from build123d import *

# Parameters (mm, degrees)
F0_W     = 609.6
F0_H     = 838.2
F1_DEPTH = 584.2
F2_DEPTH = 2.032
F3_W     = 609.6
F3_H     = 406.4
F4_DEPTH = 44.45
F5_W     = 609.6
F5_H     = 76.2
F6_DEPTH = 12.7


with BuildPart() as f1:
    # F0 (on Front) → F1 (new body)
    with BuildSketch(Plane.XZ):
        with Locations((-304.8, 419.1)):
            Rectangle(F0_W, F0_H)
    extrude(amount=-F1_DEPTH)

    # F0 (on Front) → F2 (join)
    with BuildSketch(Plane.XZ):
        Polygon((0, 838.2), (0, 0), (19.05, 0), (19.05, 857.25), (-628.65, 857.25), (-628.65, 0), (-609.6, 0), (-609.6, 838.2), align=None)
    extrude(amount=-F2_DEPTH)

    # F3 (on face) → F4 (join)
    with BuildSketch(Plane.XZ):
        with Locations((-304.8, 635)):
            Rectangle(F3_W, F3_H)
        with Locations((-304.8, 203.2)):
            Rectangle(F3_W, F3_H)
    extrude(amount=F4_DEPTH)

    # F5 (on face) → F6 (join)
    with BuildSketch(Plane(origin=(0, 0, 0), x_dir=(1, 0, 0), z_dir=(0, 0, -1))):
        with Locations((-304.8, -114.060853)):
            Rectangle(F5_W, F5_H)
        with Locations((-304.8, -331.216)):
            Rectangle(F5_W, F5_H)
    extrude(amount=F6_DEPTH)


solid = f1.part
Check sheet for the modelled part. Datum: model origin and axes. Units: mm. A direction names the side the tool comes from. Give positions to 0.01 mm unless a question says otherwise; leave off trailing zeros. Loops run counter-clockwise (first coordinate to the right, second up) from the corner with the lowest first, then second, coordinate; pieces in that order, holes last. Notation, with made-up numbers: M -13.75,89 L 6.25,89 A30 cw 6.25,122 Z; hole C 79.25,38 d11. An arc over 180 degrees is marked long. Use a Markdown table: item, result. Add a question column.
Q1. Scan lines: line 1 along X through (y, z) = (553.5, 25.5); line 2 along Z through (x, y) = (-596.5, 194); line 3 along Y through (x, z) = (-148.5, 430). Record each from-to range of solid material in increasing order. Write a range as [from, to].
Q2. Tool access check on faces 4 (the flat face through (-309, 289, 838.2)), 5 (the flat face through (-609.6, -22, 200)), 6 (the flat face through (0, 289, 407)), 7 (the flat face through (0, -22, 200)), 8 (the flat face through (-309, 222, 0)). Record the directions out of +Z, -Z, +X, -X, +Y, -Y that give a thin tool (end or side, any length) a straight path to the whole face; none if there is none.
Q3. Sectioned sample at B-B, the plane x = -283.5. Record the cut outline in (y, z), then the cut area to 3 significant figures.
Q4. Sectioned sample at D-D, the plane y = 133.5. Record the cut outline in (x, z), then the cut area to 3 significant figures.
Q5. Sectioned sample at C-C, the plane y = 493.5. Record the cut outline in (x, z), then the cut area to 3 significant figures.
Q6. Sectioned sample at A-A, the plane z = 539.5. Record the cut outline in (x, y), then the cut area to 3 significant figures.
Q7. Mould release check, pull along Z, two halves, no side actions. Record for faces 1 (the flat face through (-309, -44.45, 638)), 2 (the flat face through (-309, 475, 0)), 3 (the flat face through (-309, -22, 431.8)): pulls with the +Z half, pulls with the -Z half, needs draft (parallel to the pull), parting line crosses it, or undercut.
Q8. Go/stop test with flat-tipped pins: pin 1 (2 mm diameter, centred on x = -165.5, z = 426, fed in from -Y); pin 2 (10 mm diameter, centred on x = -350, z = -7.5, fed in from -Y); pin 3 (22 mm diameter, centred on y = -17.5, z = 204, fed in from +X). Record where each tip stops, or that it passes through.
Verdict:
| question | item | result |
|---|---|---|
| 1 | line 1 | [-609.6, 0] |
| 1 | line 2 | [0, 838.2] |
| 1 | line 3 | [0, 584.2] |
| 2 | face 4 | +Z, +X, -X, +Y |
| 2 | face 5 | +Z, -Z, -X, -Y |
| 2 | face 6 | +Z, -Z, +X, +Y |
| 2 | face 7 | +Z, -Z, +X, -Y |
| 2 | face 8 | -Z, +X, -X |
| 3 | outline | M -44.45,0 L 75.96,0 L 75.96,-12.7 L 152.16,-12.7 L 152.16,0 L 293.12,0 L 293.12,-12.7 L 369.32,-12.7 L 369.32,0 L 584.2,0 L 584.2,838.2 L 2.03,838.2 L 2.03,857.25 L 0,857.25 L 0,838.2 L -44.45,838.2 L -44.45,431.8 L 0,431.8 L 0,406.4 L -44.45,406.4 Z |
| 3 | area | 528,000 mm^2 |
| 4 | outline | M -609.6,-12.7 L 0,-12.7 L 0,838.2 L -609.6,838.2 Z |
| 4 | area | 519,000 mm^2 |
| 5 | outline | M -609.6,0 L 0,0 L 0,838.2 L -609.6,838.2 Z |
| 5 | area | 511,000 mm^2 |
| 6 | outline | M -628.65,0 L -609.6,0 L -609.6,-44.45 L 0,-44.45 L 0,0 L 19.05,0 L 19.05,2.03 L 0,2.03 L 0,584.2 L -609.6,584.2 L -609.6,2.03 L -628.65,2.03 Z |
| 6 | area | 383,000 mm^2 |
| 7 | face 1 | needs draft |
| 7 | face 2 | pulls with the -Z half |
| 7 | face 3 | undercut |
| 8 | pin 1 | y = 0 |
| 8 | pin 2 | y = 75.96 |
| 8 | pin 3 | x = 0 |
